Design review of the part built by this model. Coordinates are the model's own, in mm. A direction names the side the tool comes from. Give positions to 0.01 mm unless a question says otherwise; leave off trailing zeros. Write each loop counter-clockwise with the first axis right and the second up, starting at its lowest first coordinate (ties: lowest second). Pieces come first, ordered by that corner, then holes. Notation, with made-up numbers: (40, 41.25) -> (77, 41.25) arc R13 ccw to (77, 66.25) -> close; hole circle Ø5 at (59.5, -31). An arc over 180 degrees is marked (long way). Return JSON: item names as keys, results as strings. Group by question number.
Autodesk Fusion 360 part; units mm, degrees
sketch "Sketch1" plane through (0, 0, 0) normal (1, 0, 0) x (0, 1, 0) in component "stand"
  line L0 (-20.953, -72.187) -> (-7.2365, -34.5012)
  line L1 (-2.2234, -33.4813) -> (33.8703, -72.187)
  line L2 (-20.953, -72.187) -> (-32.2294, -68.0828)
  line L3 (-32.2294, -68.0828) -> (-30.5193, -63.3843)
  arc A0 (-2.2234, -33.4813) -> (-7.2365, -34.5012) centre (-4.4174, -35.5273) ccw
  line L4 (-4.0518, -35.1863) -> (32.042, -73.892)
  arc A1 (-4.0518, -35.1863) -> (-4.8873, -35.3562) centre (-4.4174, -35.5273) ccw
  line L5 (-19.4589, -75.3913) -> (-4.8873, -35.3562)
  line L6 (-19.4589, -75.3913) -> (-35.4336, -69.577)
  line L7 (-35.4336, -69.577) -> (-32.8685, -62.5293)
  line L8 (-32.8685, -62.5293) -> (-30.5193, -63.3843)
  line L9 (33.8703, -72.187) -> (32.042, -73.892)
  line L10 (-19.4589, -75.3913) -> (32.042, -73.892) construction
  point P0 (-20.953, -72.187)
  point P1 (-30.35, -68.7668)
  point P2 (-5.5621, -29.9009)
  dimension "d5" = 45
  dimension "d8" = 12
  dimension "d9" = 5
  dimension "d10" = 3
  dimension "d11" = 2.5
  dimension "d17" = 68.332
extrude "Extrude1" add sketch "Sketch1" along normal mid plane 50 in component "stand"
fillet "Fillet1" radius 0.5 20 edges at (25, 15.8235, -52.8342) (25, -5.0155, -32.5875) (25, -14.0948, -53.3441) (25, -12.1731, -55.3738) (25, -4.5171, -35.0373) (25, 13.9951, -54.5392) (25, -26.5912, -70.1349) (25, -34.1511, -66.0531) (25, -31.3743, -65.7336) (0, -30.5193, -63.3843) (0, -32.8685, -62.5293) (-25, 13.9951, -54.5392) (-25, -4.5171, -35.0373) (-25, -12.1731, -55.3738) (-25, -14.0948, -53.3441) (-25, -5.0155, -32.5875) (-25, 15.8235, -52.8342) (-25, -26.5912, -70.1349) (-25, -31.3743, -65.7336) (-25, -34.1511, -66.0531) in component "stand"
component "stand" placed x (1, 0, 0) y (0, 1, 0) z (0, 0, 1) at (0, 0, 0)
Q1. Insertion check: pin 1 (2 mm diameter, centred on x = 2.5, y = 12.5, fed in from +Z); pin 2 (5 mm diameter, centred on x = -17.5, y = 7, fed in from -Z); pin 3 (12 mm diameter, centred on x = 14.5, z = -62.5, fed in from +Y); pin 4 (8 mm diameter, centred on y = -15.5, z = -63.5, fed in from +X). Each pin has a flat end and moves straight along its axis. Give the tip position at first contact, or say it passes through.
Q2. For L1, parallel to Y at x = -5.5, z = -44.5; L2, parallel to Z at x = -11, y = -4.5; L3, parallel to Y at x = 1.5, z = -67.5, list the stretches that pass through material, from the lowest coordinate up. Write a range as from..to.
Q3. Take a section at A-A, the plane x = 12.5. Give the boundary of the cut face in (y, z).
Q4. Mouldability with a two-part tool opening along Z and no side actions: class faces 5 (the face through (24.86, -31.59, -65.88)), 6 (the face through (-0.34, -14.19, -53.61)), 7 (the face through (0, 33, -73)), 8 (the face through (-0.34, -31.47, -66)) as +Z half, -Z half, draft (parallel to the pull), parting line (faces both ways), or undercut.
Q5. Take a section at B-B, the plane z = -67. Count the separate pieces of the cut face and the enclosed holes in it, plus the area to 3 significant figures.
Q6. Tool access review of faces 1 (the face through (-24.8, -26.7, -70.2)), 2 (the face through (-24.85, 14.35, -54.71)), 3 (the face through (24.86, 14.36, -54.71)), 4 (the face through (24.86, -26.73, -70.25)): name each direction out of +Z, -Z, +X, -X, +Y, -Y from which nothing blocks a thin tool from reaching the whole face with its end or side.
Final values:
{
 "1": {"pin 1": "stops at z = -48.2", "pin 2": "stops at z = -49.72", "pin 3": "stops at y = 30.43", "pin 4": "stops at x = 25"},
 "2": {"L1": "y = -10.88..-8.22, 4.63..8.05", "L2": "z = -35.03..-32.53", "L3": "y = -34.68..-32.02, -19.25..-16.59, 26.08..29.5"},
 "3": {"outline": "(-35.43, -69.58) -> (-19.46, -75.39) -> (-4.89, -35.36) arc R0.5 cw to (-4.05, -35.19) -> (32.04, -73.89) -> (33.87, -72.19) -> (-2.22, -33.48) arc R3 ccw to (-7.24, -34.5) -> (-20.95, -72.19) -> (-32.23, -68.08) -> (-30.69, -63.85) arc R0.5 ccw to (-30.99, -63.21) -> (-32.4, -62.7) arc R0.5 ccw to (-33.04, -63) -> close"},
 "4": {"face 5": "undercut", "face 6": "+Z half", "face 7": "-Z half", "face 8": "undercut"},
 "5": {"separate pieces": "3", "enclosed holes": "0", "area": "436 mm²"},
 "6": {"face 1": "-X", "face 2": "-Z, -X", "face 3": "-Z, +X", "face 4": "+X"}
}
